Could you check a few things on this drawing? It's one solid part, dimensions in mm from its lowest x, y, z. A direction names the side the tool comes from. Round coordinates to 2 decimals unless told otherwise and drop trailing zeros. Write each loop counter-clockwise with the first axis right and the second up, starting at its lowest first coordinate (ties: lowest second). Pieces come first, ordered by that corner, then holes. Notation, with made-up numbers: (-21.75, 76) - (28.25, 76) arc R28 ccw to (28.25, 110) - close; hole circle Ø5 at (86, -38). An arc over 180 degrees is marked (long way). One line per question, with ' | ' between items. Start each with the question number.
(1) Will these pins go through, and if not, where does the flat tip stop? pin 1 (7.5 mm diameter, centred on y = 66, z = 13.5, fed in from -X); pin 2 (2 mm diameter, centred on x = 19.5, z = 38.5, fed in from +Y); pin 3 (14.5 mm diameter, centred on y = 44.5, z = 97, fed in from +X); pin 4 (13 mm diameter, centred on x = 30, y = 55, fed in from -Z).
(2) Thinking about a two-plate mould opening in Z: for the marked faces 5, 6, 7 and 8, which applies, pulls with the +Z half, pulls with the -Z half, needs draft (parallel to the pull), parting line crosses it, or undercut?
(3) If I drill on L1, parallel to Y at x = 30, z = 94; L2, parallel to Z at x = 19.5, y = 32; L3, parallel to Y at x = 23, z = 38.5, over which ranges is the centre line in solid material (lowest first)?
(4) Imagine slicing it at B-B (y = 61). Write out the boundary of the cut face in (x, z), plus the area to 3 significant figures.
(5) For the marked faces 1, 2, 3 and 4, which set-ups out of +Z, -Z, +X, -X, +Y, -Y let a thin tool reach every point of the face, with its end or its side?
(6) Imagine slicing it at D-D (x = 53). Write out the boundary of the cut face in (y, z).
(7) Imagine slicing it at C-C (z = 92.5). Write out the boundary of the cut face in (x, y), plus the area to 3 significant figures.
(8) Imagine slicing it at A-A (x = 30). Write out the boundary of the cut face in (y, z).
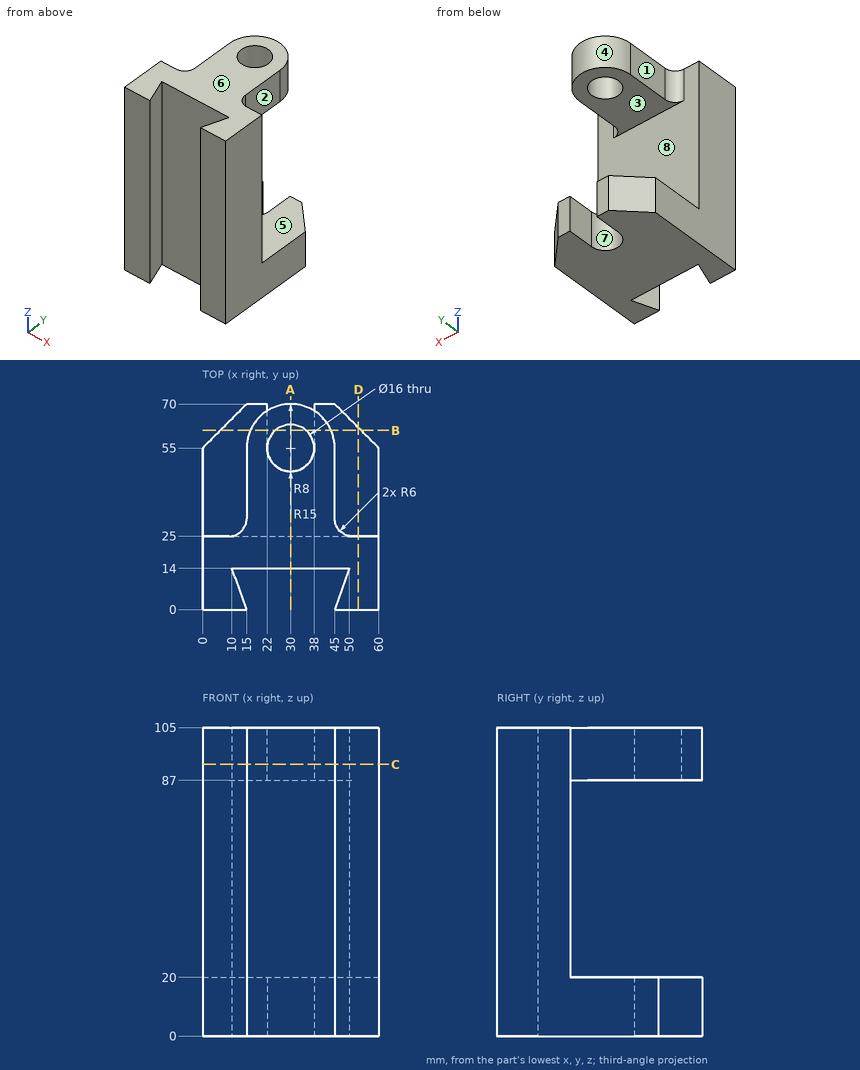
Check sheet entries:
1) pin 1: x = 7.25 | pin 2: y = 25 | pin 3: x = 45 | pin 4: through
2) face 5: undercut | face 6: pulls with the +Z half | face 7: needs draft | face 8: undercut
3) L1: 14 to 47, 63 to 70 | L2: 0 to 20, 87 to 105 | L3: 14 to 25
4) outline: (6, 0) - (22, 0) - (22, 20) - (6, 20) - close; (16.25, 87) - (24.71, 87) - (24.71, 105) - (16.25, 105) - close; (35.29, 87) - (43.75, 87) - (43.75, 105) - (35.29, 105) - close; (38, 0) - (54, 0) - (54, 20) - (38, 20) - close | area: 944 mm^2
5) face 1: +Z, -X, +Y | face 2: +Z, +X, +Y | face 3: +X, -X, +Y | face 4: +Z, +Y
6) outline: (0, 0) - (62, 0) - (62, 20) - (25, 20) - (25, 105) - (0, 105) - close
7) outline: (0, 0) - (15, 0) - (10, 14) - (50, 14) - (45, 0) - (60, 0) - (60, 25) - (51, 25) arc R6 cw to (45, 31) - (45, 55) arc R15 ccw to (15, 55) - (15, 31) arc R6 cw to (9, 25) - (0, 25) - close; hole circle Ø16 at (30, 55) | area: 2,080 mm^2
8) outline: (14, 0) - (47, 0) - (47, 20) - (25, 20) - (25, 87) - (47, 87) - (47, 105) - (14, 105) - close; (63, 87) - (70, 87) - (70, 105) - (63, 105) - close
